Autodesk Inventor part; units mm, degrees
ref_plane "YZ Plane" through (0, 0, 0) normal (1, 0, 0) x (0, 1, 0)
ref_plane "XZ Plane" through (0, 0, 0) normal (0, 1, 0) x (-1, 0, 0)
ref_plane "XY Plane" through (0, 0, 0) normal (0, 0, 1) x (1, 0, 0)
sketch "Sketch1" plane through (0, 0, 0) normal (0, 1, 0) x (-1, 0, 0)
  circle A0 centre (0, 0) radius 40
  circle A1 centre (0, 0) radius 46
  circle A2 centre (0, 0) radius 37
  circle A3 centre (0, 0) radius 49
  line L0 (-46, 0) -> (-49, 0)
  line L1 (0, 0) -> (-46.7041, -14.8233)
  point P0 (-43.8446, -13.9157)
  dimension "d0" = 80
  dimension "d1" = 6
  dimension "d2" = 3
  dimension "d7" = 3
  dimension "d8" = 15
extrude "Extrusion1" add sketch "Sketch1" along normal blind 23 contours A0
extrude "Extrusion2" add sketch "Sketch1" along normal blind 3 contours A1
extrude "Extrusion3" add sketch "Sketch1" along normal up to surface (23 mm away) contours L1 A3 L0 A1 picked at (-46.1746, -12.9028)
properties part number "80mm-CoilForm_3DPrint"
Geometry: final body of the model. Coordinates: model frame, mm. A direction names the side the tool comes from. Round coordinates to 2 decimals unless told otherwise and drop trailing zeros. Order: outer loops, then holes, each group sorted by start corner. A loop starts at its lowest first (then second) coordinate and runs counter-clockwise, first axis right, second up. Notation, with made-up numbers: (61.5, 22) - (89.5, 22) arc R16 ccw to (89.5, 41) - close; hole circle Ø6 at (68.5, 34). An arc over 180 degrees is marked (long way). Write each question's results on one line, items separated by ' | '.
Item 1: Mould query, pull axis Z, two halves, no side actions, for faces 6 (the flat face through (47, 23, -7)), 7 (the cylindrical face through (8.02, 11.34, 36.12)), 8 (the cylindrical face through (-45.124, 1.479, 8.936)). Classes: pulls with the +Z half, pulls with the -Z half, needs draft (parallel to the pull), parting line crosses it, or undercut.
Completed:
face 6: needs draft | face 7: undercut | face 8: parting line crosses it
Item 2: Section C-C, the plane y = 1.75. Return the cut outline in (x, z), and give its area (3 significant figures).
Completed:
outline: (43.84, -13.92) - (46.7, -14.82) arc R49 ccw to (49, 0) - (46, 0) arc R46 ccw (long way) to start; hole circle Ø74 at (0, 0) | area: 2,390 mm^2
Item 3: Section A-A, the plane y = 11.75. Return the cut outline in (x, z).
Completed:
outline: circle Ø80 at (0, 0); (43.84, -13.92) - (46.7, -14.82) arc R49 ccw to (49, 0) - (46, 0) arc R46 cw to start; hole circle Ø74 at (0, 0)
Item 4: Section D-D, the plane z = 20. Return the cut outline in (x, y).
Completed:
outline: (-41.42, 0) - (-31.13, 0) - (-31.13, 23) - (-34.64, 23) - (-34.64, 3) - (-41.42, 3) - close; (31.13, 0) - (41.42, 0) - (41.42, 3) - (34.64, 3) - (34.64, 23) - (31.13, 23) - close
Item 5: Material intervals for line 1 along X through (y, z) = (15.75, -0.5); line 2 along Z through (x, y) = (0, 7.25); line 3 along X through (y, z) = (5.5, -8), sorted ascending. Write a range as [from, to].
Completed:
line 1: [-40, -37], [37, 40], [46, 49] | line 2: [-40, -37], [37, 40] | line 3: [-39.19, -36.12], [36.12, 39.19], [45.3, 48.34]
Item 6: Reachability of faces 1 (the cylindrical face through (48.406, 11.339, -7.604)), 2 (the flat face through (45.25, 11.34, -14.36)), 3 (the cylindrical face through (8.67, 12.86, 39.05)), 4 (the flat face through (47, 11, 0)), 5 (the cylindrical face through (45.443, 12.86, -7.139)) from +Z, -Z, +X, -X, +Y, -Y: full face, straight path, thin tool, end or side. Return the list, or none.
Completed:
face 1: -Z, +X, +Y, -Y | face 2: -Z, +Y, -Y | face 3: +Y | face 4: +Z, +X, +Y, -Y | face 5: +Z, +Y
Item 7: Section B-B, the plane x = 0. Return the cut outline in (y, z), and give its area (3 significant figures).
Completed:
outline: (0, -46) - (3, -46) - (3, -40) - (23, -40) - (23, -37) - (0, -37) - close; (0, 37) - (23, 37) - (23, 40) - (3, 40) - (3, 46) - (0, 46) - close | area: 174 mm^2
Item 8: First-contact query: pin 1 Ø5 at (y, z) = (4, 2.5) entering from -X; pin 2 Ø3 at (y, z) = (16, 3.5) entering from -X; pin 3 Ø0.9 at (x, y) = (47.5, 11) entering from +Z; pin 4 Ø1.5 at (y, z) = (17.5, -24) entering from -X. Flat tips, straight axial feed; report the tip coordinate or a pass-through.
Completed:
pin 1: x = -46 | pin 2: x = -39.95 | pin 3: z = 0 | pin 4: x = -32.55
